Read the model definition and answer for the solid it produces. Units are mm, in the model's axes. A direction names the side the tool comes from. Coordinates: 2 decimals unless noted, no trailing zeros. Loops run counter-clockwise (first coordinate to the right, second up) from the corner with the lowest first, then second, coordinate; pieces in that order, holes last.
from build123d import *

# Parameters (mm, degrees)
SKETCH_1_W          = 50
SKETCH_1_H          = 50
EXTRUDE_1_DEPTH     = 20
SKETCH_2_R          = 2
CUT_EXTRUDE_1_DEPTH = 20
CUT_EXTRUDE_2_DEPTH = 20
FILLET_1_R          = 5


with BuildPart() as part:
    # 草图1 → 凸台-拉伸1 (new body)
    with BuildSketch(Plane(origin=(0, 0, 0), x_dir=(1, 0, 0), z_dir=(0, 1, 0))):
        with Locations((25, -25)):
            Rectangle(SKETCH_1_W, SKETCH_1_H)
    extrude(amount=EXTRUDE_1_DEPTH)

    # 草图2 → 切除-拉伸1 (cut)
    with BuildSketch(Plane(origin=(0, 20, 0), x_dir=(1, 0, 0), z_dir=(0, 1, 0))):
        with Locations(Location((5, -3.945505115, 0), (0, 0, 270))):
            Circle(SKETCH_2_R)
        with Locations(Location((45, -3.945505115, 0), (0, 0, 270))):
            Circle(SKETCH_2_R)
        with Locations(Location((5, -43.945505115, 0), (0, 0, 270))):
            Circle(SKETCH_2_R)
        with Locations(Location((45, -43.945505115, 0), (0, 0, 270))):
            Circle(SKETCH_2_R)
    extrude(amount=-CUT_EXTRUDE_1_DEPTH, mode=Mode.SUBTRACT)

    # 草图3 → 切除-拉伸2 (cut)
    with BuildSketch(Plane(origin=(0, 20, 0), x_dir=(1, 0, 0), z_dir=(0, 1, 0))):
        with BuildLine():
            Line((25, -23.155221491), (25, -4.579448382))
            ThreePointArc((25, -4.579448382), (29.544000218, -5.091434245), (33.860145291, -6.601718727))
            Line((33.860145291, -6.601718727), (25.800419398, -23.337911995))
            ThreePointArc((25.800419398, -23.337911995), (25.410501837, -23.201473939), (25, -23.155221491))
        make_face()
        with BuildLine():
            Line((26.442305917, -23.849799413), (40.965430144, -12.267994318))
            ThreePointArc((40.965430144, -12.267994318), (43.398281273, -16.139854709), (44.908565755, -20.455999782))
            Line((44.908565755, -20.455999782), (26.798526061, -24.589498163))
            ThreePointArc((26.798526061, -24.589498163), (26.662088005, -24.199580602), (26.442305917, -23.849799413))
        make_face()
        with BuildLine():
            Line((26.798526061, -25.410501837), (44.908565755, -29.544000218))
            ThreePointArc((44.908565755, -29.544000218), (43.398281273, -33.860145291), (40.965430144, -37.732005682))
            Line((40.965430144, -37.732005682), (26.442305917, -26.150200587))
            ThreePointArc((26.442305917, -26.150200587), (26.662088005, -25.800419398), (26.798526061, -25.410501837))
        make_face()
        with BuildLine():
            Line((25.800419398, -26.662088005), (33.860145291, -43.398281273))
            ThreePointArc((33.860145291, -43.398281273), (29.544000218, -44.908565755), (25, -45.420551618))
            Line((25, -45.420551618), (25, -26.844778509))
            ThreePointArc((25, -26.844778509), (25.410501837, -26.798526061), (25.800419398, -26.662088005))
        make_face()
        with BuildLine():
            Line((24.199580602, -26.662088005), (16.139854709, -43.398281273))
            ThreePointArc((16.139854709, -43.398281273), (12.267994318, -40.965430144), (9.034569856, -37.732005682))
            Line((9.034569856, -37.732005682), (23.557694083, -26.150200587))
            ThreePointArc((23.557694083, -26.150200587), (23.849799413, -26.442305917), (24.199580602, -26.662088005))
        make_face()
        with BuildLine():
            Line((23.201473939, -25.410501837), (5.091434245, -29.544000218))
            ThreePointArc((5.091434245, -29.544000218), (4.579448382, -25), (5.091434245, -20.455999782))
            Line((5.091434245, -20.455999782), (23.201473939, -24.589498163))
            ThreePointArc((23.201473939, -24.589498163), (23.155221491, -25), (23.201473939, -25.410501837))
        make_face()
        with BuildLine():
            Line((23.557694083, -23.849799413), (9.034569856, -12.267994318))
            ThreePointArc((9.034569856, -12.267994318), (12.267994318, -9.034569856), (16.139854709, -6.601718727))
            Line((16.139854709, -6.601718727), (24.199580602, -23.337911995))
            ThreePointArc((24.199580602, -23.337911995), (23.849799413, -23.557694083), (23.557694083, -23.849799413))
        make_face()
    extrude(amount=-CUT_EXTRUDE_2_DEPTH, mode=Mode.SUBTRACT)

    # 圆角1
    fillet_1_edges = [part.edges().sort_by_distance(p)[0] for p in [
        (0, 10, 0),
        (50, 10, 0),
        (50, 10, 50),
        (0, 10, 50),
    ]]
    fillet(fillet_1_edges, radius=FILLET_1_R)


solid = part.part
Item 1: Which of the six approach directions +Z, -Z, +X, -X, +Y, -Y give full straight-line access (tool end or side, diameter ignored) to faces 5 (the face through (1, 10, 48)), 6 (the face through (14.02, 10.14, 22.494))?
Numbers:
face 5: +Z, -X, +Y, -Y
face 6: +Y, -Y
Item 2: A cutting plane is placed at C-C on x = 12. Determine the outline of the cut face in (y, z), then the cut area to 3 significant figures.
Numbers:
outline: (0, 0) - (20, 0) - (20, 9.25) - (0, 9.25) - close; (0, 14.63) - (20, 14.63) - (20, 22.03) - (0, 22.03) - close; (0, 27.97) - (20, 27.97) - (20, 35.37) - (0, 35.37) - close; (0, 40.75) - (20, 40.75) - (20, 50) - (0, 50) - close
area: 666 mm2
Item 3: A cutting plane is placed at D-D on y = 16. Give the number of separate pieces and of enclosed holes in the cut face, then the cut area to 3 significant figures.
Numbers:
separate pieces: 1
enclosed holes: 11
area: 1,780 mm2
Item 4: Given pin 1 (3 mm diameter, centred on x = 19, z = 5.5, fed in from -Y), flat-ended and moving along its own axis, determine where the tip first touches the part or whether it passes through.
Numbers:
pin 1: stops at y = 0
Item 5: A cutting plane is placed at A-A on x = 37. Determine the outline of the cut face in (y, z), then the cut area to 3 significant figures.
Numbers:
outline: (0, 0) - (20, 0) - (20, 15.43) - (0, 15.43) - close; (0, 22.26) - (20, 22.26) - (20, 27.74) - (0, 27.74) - close; (0, 34.57) - (20, 34.57) - (20, 50) - (0, 50) - close
area: 727 mm2
Item 6: A cutting plane is placed at B-B on z = 14.5. Determine the outline of the cut face in (x, y).
Numbers:
outline: (0, 0) - (11.83, 0) - (11.83, 20) - (0, 20) - close; (19.94, 0) - (25, 0) - (25, 20) - (19.94, 20) - close; (30.06, 0) - (38.17, 0) - (38.17, 20) - (30.06, 20) - close; (42.51, 0) - (50, 0) - (50, 20) - (42.51, 20) - close
Item 7: Determine the mould class of faces 1 (the face through (29.89, 10.14, 14.85)), 2 (the face through (12.318, 10.14, 41.005)), 3 (the face through (48, 10, 49)), 4 (the face through (25, 0, 25)) for opening direction X: released by +X, released by -X, zero draft, split by the parting line, or undercut.
Numbers:
face 1: undercut
face 2: undercut
face 3: released by +X
face 4: zero draft
Item 8: Find the intervals of material crossed by line 1 along X through (y, z) = (6.75, 34); line 2 along X through (y, z) = (14.25, 43.5); line 3 along X through (y, z) = (15.75, 4), in increasing order.
Numbers:
line 1: x = 0 to 13.71, 20.67 to 25, 29.33 to 36.29, 43.33 to 50
line 2: x = 0 to 3.05, 6.95 to 25, 33.65 to 43.05, 46.95 to 50
line 3: x = 0.1 to 3, 7 to 43, 47 to 49.9
